from build123d import *

# Parameters (mm, degrees)
SKIZZE5_R                       = 2.85
AUFSATZ_LINEAR_AUSTRAGEN2_DEPTH = 2
SKIZZE7_R                       = 1.5
SKIZZE7_R_2                     = 2.5
SCHNITT_LINEAR_AUSTRAGEN1_DEPTH = 2
SKIZZE8_W                       = 11
SKIZZE8_H                       = 32.890928956
AUFSATZ_LINEAR_AUSTRAGEN3_DEPTH = 2
SKIZZE9_W                       = 13
SKIZZE9_H                       = 20.072612556
SCHNITT_LINEAR_AUSTRAGEN2_DEPTH = 2
SKIZZE10_R                      = 3.4
AUFSATZ_LINEAR_AUSTRAGEN4_DEPTH = 2
SKIZZE11_R                      = 1.5
SCHNITT_LINEAR_AUSTRAGEN3_DEPTH = 5
VERRUNDUNG3_R                   = 3
VERRUNDUNG4_R                   = 3
VERRUNDUNG5_R                   = 3
VERRUNDUNG6_R                   = 3
SKIZZE12_W                      = 4.557802571
SKIZZE12_H                      = 1.72453781
SKIZZE12_W_2                    = 7.81907696
SKIZZE12_H_2                    = 1.295060399
SKIZZE12_W_3                    = 1.755726722
SKIZZE12_H_3                    = 5.084854061
SKIZZE12_H_4                    = 4.524687863
SCHNITT_LINEAR_AUSTRAGEN4_DEPTH = 10


with BuildPart() as part:
    # Skizze5 → Aufsatz-Linear austragen2 (new body)
    with BuildSketch(Plane.XY):
        with BuildLine():
            Line((-40.726132402, -24.649552882), (-40.726132402, 23.890447118))
            ThreePointArc((-40.726132402, 23.890447118), (-44.126132402, 20.490447118), (-47.526132402, 23.890447118))
            Line((-47.526132402, 23.890447118), (-47.526132402, -24.649552882))
            ThreePointArc((-47.526132402, -24.649552882), (-44.126132402, -21.249552882), (-40.726132402, -24.649552882))
        make_face()
        with BuildLine():
            Line((-40.726132402, 23.890447118), (-40.775983963, 24.470537999))
            ThreePointArc((-40.775983963, 24.470537999), (-44.126132402, 27.290447118), (-47.476280842, 24.470537999))
            Line((-47.476280842, 24.470537999), (-47.526132402, 23.890447118))
            ThreePointArc((-47.526132402, 23.890447118), (-44.126132402, 20.490447118), (-40.726132402, 23.890447118))
        make_face()
        with Locations((-44.126132402, 30.290447118)):
            Circle(SKIZZE5_R)
        with BuildLine():
            Line((-40.775983963, 24.470537999), (-41.276132402, 30.290447118))
            ThreePointArc((-41.276132402, 30.290447118), (-44.126132402, 27.440447118), (-46.976132402, 30.290447118))
            Line((-46.976132402, 30.290447118), (-47.476280842, 24.470537999))
            ThreePointArc((-47.476280842, 24.470537999), (-44.126132402, 27.290447118), (-40.775983963, 24.470537999))
        make_face()
        with BuildLine():
            Line((-40.775983963, -25.229643764), (-40.726132402, -24.649552882))
            ThreePointArc((-40.726132402, -24.649552882), (-44.126132402, -21.249552882), (-47.526132402, -24.649552882))
            Line((-47.526132402, -24.649552882), (-47.476280842, -25.229643764))
            ThreePointArc((-47.476280842, -25.229643764), (-44.126132402, -28.049552882), (-40.775983963, -25.229643764))
        make_face()
        with BuildLine():
            Line((-41.276132402, -31.049552882), (-40.775983963, -25.229643764))
            ThreePointArc((-40.775983963, -25.229643764), (-44.126132402, -28.049552882), (-47.476280842, -25.229643764))
            Line((-47.476280842, -25.229643764), (-46.976132402, -31.049552882))
            ThreePointArc((-46.976132402, -31.049552882), (-44.126132402, -28.199552882), (-41.276132402, -31.049552882))
        make_face()
        with Locations((-44.126132402, -31.049552882)):
            Circle(SKIZZE5_R)
    extrude(amount=AUFSATZ_LINEAR_AUSTRAGEN2_DEPTH)

    # Skizze7 → Schnitt-Linear austragen1 (cut)
    with BuildSketch(Plane(origin=(0, 0, 0), x_dir=(-1, 0, 0), z_dir=(0, 0, -1))):
        with Locations((44.126132402, 30.290447118)):
            Circle(SKIZZE7_R)
        with Locations((44.126132402, 23.890447118)):
            Circle(SKIZZE7_R_2)
        with Locations((44.126132402, -24.649552882)):
            Circle(SKIZZE7_R_2)
        with Locations((44.126132402, -31.049552882)):
            Circle(SKIZZE7_R)
    extrude(amount=-SCHNITT_LINEAR_AUSTRAGEN1_DEPTH, mode=Mode.SUBTRACT)

    # Skizze8 → Aufsatz-Linear austragen3 (add)
    with BuildSketch(Plane(origin=(0, 0, 0), x_dir=(-1, 0, 0), z_dir=(0, 0, -1))):
        with Locations((53.026132402, -0.786592511)):
            Rectangle(SKIZZE8_W, SKIZZE8_H)
    extrude(amount=-AUFSATZ_LINEAR_AUSTRAGEN3_DEPTH)

    # Skizze9 → Schnitt-Linear austragen2 (cut)
    with BuildSketch(Plane(origin=(0, 0, 0), x_dir=(-1, 0, 0), z_dir=(0, 0, -1))):
        with Locations((47.226132402, -0.610696343)):
            Rectangle(SKIZZE9_W, SKIZZE9_H)
    extrude(amount=-SCHNITT_LINEAR_AUSTRAGEN2_DEPTH, mode=Mode.SUBTRACT)

    # Skizze10 → Aufsatz-Linear austragen4 (add)
    with BuildSketch(Plane(origin=(0, 0, 0), x_dir=(-1, 0, 0), z_dir=(0, 0, -1))):
        with Locations((44.126132402, 23.890447118)):
            Circle(SKIZZE10_R)
        with Locations((44.126132402, -24.649552882)):
            Circle(SKIZZE10_R)
    extrude(amount=-AUFSATZ_LINEAR_AUSTRAGEN4_DEPTH)

    # Skizze11 → Schnitt-Linear austragen3 (cut)
    with BuildSketch(Plane(origin=(0, 0, 0), x_dir=(-1, 0, 0), z_dir=(0, 0, -1))):
        with Locations((44.126132402, -24.649552882)):
            Circle(SKIZZE11_R)
        with Locations((44.126132402, 23.890447118)):
            Circle(SKIZZE11_R)
    extrude(amount=-SCHNITT_LINEAR_AUSTRAGEN3_DEPTH, mode=Mode.SUBTRACT)

    # Verrundung3
    verrundung3_edges = [part.edges().sort_by_distance(p)[0] for p in [
        (-40.726132402, 9.425609935, 1),
        (-53.726132402, 9.425609935, 1),
    ]]
    fillet(verrundung3_edges, radius=VERRUNDUNG3_R)

    # Verrundung4
    verrundung4_edges = [part.edges().sort_by_distance(p)[0] for p in [
        (-40.726132402, -10.647002621, 1),
        (-53.726132402, -10.647002621, 1),
    ]]
    fillet(verrundung4_edges, radius=VERRUNDUNG4_R)

    # Verrundung5
    verrundung5_edges = [part.edges().sort_by_distance(p)[0] for p in [
        (-47.526132402, -17.232056989, 1),
        (-58.526132402, -17.232056989, 1),
    ]]
    fillet(verrundung5_edges, radius=VERRUNDUNG5_R)

    # Verrundung6
    verrundung6_edges = [part.edges().sort_by_distance(p)[0] for p in [
        (-47.526132402, 15.658871967, 1),
        (-58.526132402, 15.658871967, 1),
    ]]
    fillet(verrundung6_edges, radius=VERRUNDUNG6_R)

    # Skizze12 → Schnitt-Linear austragen4 (cut)
    with BuildSketch(Plane(origin=(0, 0, 0), x_dir=(-1, 0, 0), z_dir=(0, 0, -1))):
        with Locations((44.015184194, 33.533655536)):
            Rectangle(SKIZZE12_W, SKIZZE12_H)
        with Locations((44.191445116, -33.911577792)):
            Rectangle(SKIZZE12_W_2, SKIZZE12_H_2)
        with Locations((40.756736433, 29.933182837)):
            Rectangle(SKIZZE12_W_3, SKIZZE12_H_3)
        with Locations((40.756736433, -30.635891291)):
            Rectangle(SKIZZE12_W_3, SKIZZE12_H_4)
    extrude(amount=-SCHNITT_LINEAR_AUSTRAGEN4_DEPTH, mode=Mode.SUBTRACT)


solid = part.part
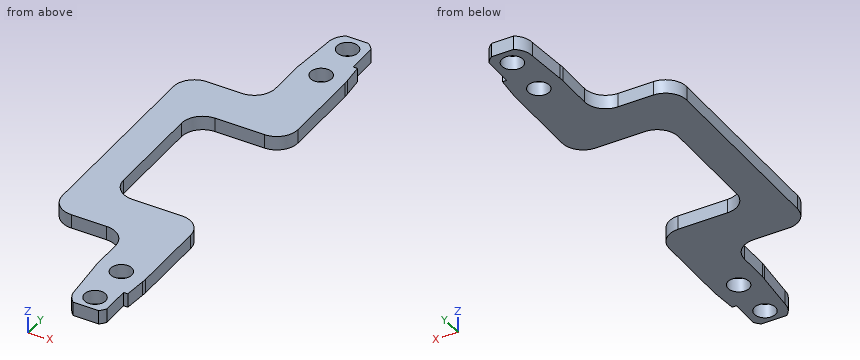
Check sheet for the modelled part. Datum: model origin and axes. Units: mm. Coordinates: 2 decimals unless noted, no trailing zeros. Write each loop counter-clockwise with the first axis right and the second up, starting at its lowest first coordinate (ties: lowest second). Pieces come first, ordered by that corner, then holes. Notation, with made-up numbers: M 64,5 L 119,5 A29 ccw 119,31 Z; hole C 29,-40 d8. An arc over 180 degrees is marked long. Answer as CSV lines item,"result".
Q1. Cross-section at C-C (z = 0.75). Count the separate pieces of the cut face and the enclosed holes in it, then the cut area to 3 significant figures.
Check result:
separate pieces,"1"
enclosed holes,"4"
area,"502 mm^2"
Q2. Cross-section at A-A (x = -51.75). Record the boundary of the cut face in (y, z).
Check result:
outline,"M -17.23,0 L -10.47,0 L -10.47,2 L -17.23,2 Z; M 9.25,0 L 15.66,0 L 15.66,2 L 9.25,2 Z"
Q3. Go/stop test with flat-tipped pins: pin 1 (0.6 mm diameter, centred on y = -23, z = 1, fed in from -X); pin 2 (0.5 mm diameter, centred on x = -41.5, z = 1, fed in from -Y); pin 3 (1 mm diameter, centred on x = -52.5, z = 1.5, fed in from -Y); pin 4 (2.5 mm diameter, centred on x = -44.13, y = 23.89, fed in from +Z). Record where each tip stops, or that it passes through.
Check result:
pin 1,"x = -47.53"
pin 2,"y = -32.62"
pin 3,"y = -17.23"
pin 4,"through"
Q4. Cross-section at B-B (y = -24). Record the boundary of the cut face in (x, z), then the cut area to 3 significant figures.
Check result:
outline,"M -47.53,0 L -45.48,0 L -45.48,2 L -47.53,2 Z; M -42.77,0 L -40.73,0 L -40.73,2 L -42.77,2 Z"
area,"8.19 mm^2"
Q5. Material ranges on probe 1 along Y at (x, z) = (-44.25, 1.3); probe 2 along X at (y, z) = (24, 0.5); probe 3 along Y at (x, z) = (-50.25, 1.85), recorded low to high. Write a range as from..to.
Check result:
probe 1,"-33.26..-32.54, -29.55..-26.14, -23.15..-10.65, 9.43..22.4, 25.39..28.8, 31.79..32.67"
probe 2,"-47.52..-45.62, -42.63..-40.73"
probe 3,"-17.24..-10.65, 9.43..15.67"
Q6. Cross-section at D-D (y = -5). Record the boundary of the cut face in (x, z), then the cut area to 3 significant figures.
Check result:
outline,"M -58.53,0 L -53.73,0 L -53.73,2 L -58.53,2 Z"
area,"9.60 mm^2"
